from build123d import *

# Parameters (mm, degrees)
F1_DEPTH = 16.5
F2_R     = 2
F3_R     = 3
F4_DEPTH = 25
F5_R     = 3
F6_DEPTH = 25


with BuildPart() as f1:
    # F0 (on Front) → F1 (new body)
    with BuildSketch(Plane.XZ):
        Polygon((5, 0), (0, 0), (0, -5), (0, -150), (5, -150), (5, -5), (150, -5), (150, 0), align=None)
    extrude(amount=F1_DEPTH)

    # F2
    f2_edges = [f1.edges().sort_by_distance(p)[0] for p in [
        (5, -8.25, -5),
        (150, -8.25, -5),
        (5, -8.25, -150),
    ]]
    fillet(f2_edges, radius=F2_R)

    # F3 (on face) → F4 (cut)
    with BuildSketch(Plane(origin=(0, 0, -5), x_dir=(1, 0, 0), z_dir=(0, 0, -1))):
        with Locations((133, 8.25)):
            Circle(F3_R)
        with Locations((22, 8.25)):
            Circle(F3_R)
    extrude(amount=-F4_DEPTH, mode=Mode.SUBTRACT)

    # F5 (on face) → F6 (cut)
    with BuildSketch(Plane.YZ.offset(5)):
        with Locations((-8.25, -133)):
            Circle(F5_R)
        with Locations((-8.25, -22)):
            Circle(F5_R)
    extrude(amount=-F6_DEPTH, mode=Mode.SUBTRACT)


solid = f1.part
Geometry: final body of the model. Coordinates: model frame, mm. A direction names the side the tool comes from. Give positions to 0.01 mm unless a question says otherwise; leave off trailing zeros. Write each loop counter-clockwise with the first axis right and the second up, starting at its lowest first coordinate (ties: lowest second). Pieces come first, ordered by that corner, then holes.
(1) Cut plane D-D, the plane x = 76. Return loops of the section in (y, z), then the cut area to 3 significant figures.
(2) Cut plane B-B, the plane x = 22. Return loops of the section in (y, z), then the cut area to 3 significant figures.
(3) Cut plane C-C, the plane z = -133. Return loops of the section in (x, y), then the cut area to 3 significant figures.
(4) Access query for faces 4 (the flat face through (5, -8, -78)), 5 (the cylindrical face through (135.86, -9.15, -2.54)). Directions: +Z, -Z, +X, -X, +Y, -Y. A direction counts if a zero-diameter tool reaches every point of the face in a straight line with its end or side. Return the directions, or none.
(5) Ray query, line 1 (Z direction, x = 1.75, y = -8.25); line 2 (X direction, y = -8.25, z = -1.8); line 3 (Y direction, x = 133, z = -1.9). Return the intervals inside material, ascending.
(6) Cut plane A-A, the plane y = -8.25. Return loops of the section in (x, z).
(7) First-contact query: P1, Ø1, axis at x = 35.5, y = -9.5, coming from the -Z side; P2, Ø8, axis at y = -11.5, z = -90, coming from the +X side. Flat tips, straight axial feed; report the tip coordinate or a pass-through.
(8) Mould query, pull axis Y, two halves, no side actions, for faces 1 (the cylindrical face through (19.003, -8.382, -2.535)), 2 (the flat face through (2, -16.5, -41)), 3 (the flat face through (76, -8, 0)). Classes: released by +Y, released by -Y, zero draft, split by the parting line, or undercut.
Values follow:
1. outline: (-16.5, -5) - (0, -5) - (0, 0) - (-16.5, 0) - close
1. area: 82.5 mm2
2. outline: (-16.5, -5) - (-11.25, -5) - (-11.25, 0) - (-16.5, 0) - close; (-5.25, -5) - (0, -5) - (0, 0) - (-5.25, 0) - close
2. area: 52.5 mm2
3. outline: (0, -16.5) - (5, -16.5) - (5, -11.25) - (0, -11.25) - close; (0, -5.25) - (5, -5.25) - (5, 0) - (0, 0) - close
3. area: 52.5 mm2
4. face 4: -Z, +X, +Y, -Y
4. face 5: +Z, -Z
5. line 1: z = -150 to -136, -130 to -25, -19 to 0
5. line 2: x = 0 to 19, 25 to 130, 136 to 150
5. line 3: y = -16.5 to -11.25, -5.25 to 0
6. outline: (0, -150) - (3, -150) arc R2 ccw to (5, -148) - (5, -136) - (0, -136) - close; (0, -130) - (5, -130) - (5, -25) - (0, -25) - close; (0, -19) - (5, -19) - (5, -7) arc R2 cw to (7, -5) - (19, -5) - (19, 0) - (0, 0) - close; (25, -5) - (130, -5) - (130, 0) - (25, 0) - close; (136, -5) - (148, -5) arc R2 ccw to (150, -3) - (150, 0) - (136, 0) - close
7. P1: stops at z = -5
7. P2: stops at x = 5
8. face 1: undercut
8. face 2: released by -Y
8. face 3: zero draft
